Design review of the part built by this model. Coordinates are the model's own, in mm. Face numbers are marked on the shaded views. Coordinates: 2 decimals unless noted, no trailing zeros. Order: outer loops, then holes, each group sorted by start corner. A loop starts at its lowest first (then second) coordinate and runs counter-clockwise, first axis right, second up. Notation, with made-up numbers: (-32, 41) - (15, 41) arc R32 cw to (15, 77) - close; hole circle Ø1 at (52.25, 33). An arc over 180 degrees is marked (long way). Write each question's results on one line, items separated by ' | '. Start each with the question number.
```python
from build123d import *

# Parameters (mm, degrees)
SKETCH_1_R         = 30
SKETCH_1_R_2       = 23.5
EXTRUDE_1_DEPTH    = 10
SKETCH_2_R         = 31.5
SKETCH_2_R_2       = 30
EXTRUDE_2_DEPTH    = 2
HOLE_WIZARD_M4_1_D = 3.3


with BuildPart() as part:
    # 草图1 → 凸台-拉伸1 (new body)
    with BuildSketch(Plane(origin=(0, 0, 0), x_dir=(1, 0, 0), z_dir=(0, 1, 0))):
        Circle(SKETCH_1_R)
        Circle(SKETCH_1_R_2, mode=Mode.SUBTRACT)
    extrude(amount=EXTRUDE_1_DEPTH)

    # 草图2 → 凸台-拉伸2 (add)
    with BuildSketch(Plane(origin=(0, 10, 0), x_dir=(1, 0, 0), z_dir=(0, 1, 0))):
        Circle(SKETCH_2_R)
        Circle(SKETCH_2_R_2, mode=Mode.SUBTRACT)
    extrude(amount=-EXTRUDE_2_DEPTH)

    # M4 螺纹孔1 (through all)
    with Locations(Plane(origin=(-18.561553006, 0, 18.561553006), x_dir=(0, 0, -1), z_dir=(0, -1, 0))):
        with Locations((0, 0), (-7.688446994, 18.561553006), (18.561553006, -7.688446994), (37.123106012, 0), (44.811553006, 18.561553006), (37.123106012, 37.123106012), (18.561553006, 44.811553006), (0, 37.123106012)):
            Hole(HOLE_WIZARD_M4_1_D / 2)


solid = part.part
```
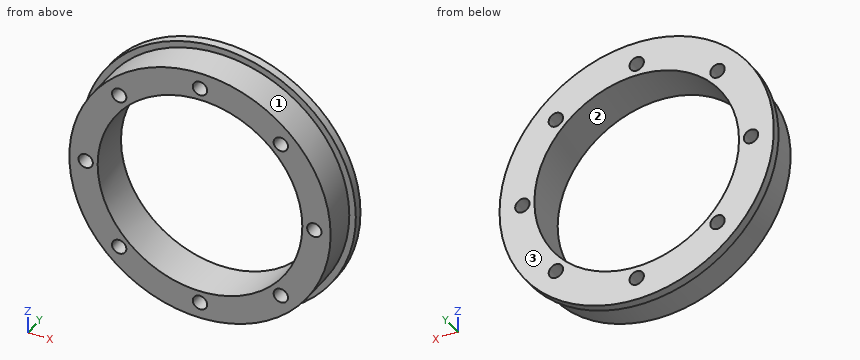
(1) Take a section at B-B (x = 0). State the section outline as (y, z) points.
(2) Mouldability with a two-part tool opening along Z and no side actions: class the marked faces 1, 2 and 3 as +Z half, -Z half, draft (parallel to the pull), parting line (faces both ways), or undercut.
(3) Clearance check with flat-ended pins moving along their axes: pin 1 (12 mm diameter, centred on x = 8.5, z = -16, fed in from +Y); pin 2 (6 mm diameter, centred on y = 2.5, z = -16.5, fed in from +X); pin 3 (6 mm diameter, centred on x = 10, y = 1, fed in from +Z); pin 4 (1 mm diameter, centred on x = 0.5, y = 5, fed in from -Z). State where each tip first meets the part, or that it passes through.
(4) Take a section at A-A (z = 0). State the section outline as (x, y) points.
(5) To check wall thickness, follow line 1 along X through (y, z) = (4.25, 0); line 2 along X through (y, z) = (2, -1); line 3 along X through (y, z) = (3.25, -21). State the ranges of each line that lie inside material, in increasing order. Write a range as [from, to].
(6) Take a section at D-D (z = -26.25). State the section outline as (x, y) points, plus the area to 3 significant figures.
(7) Take a section at C-C (x = -16). State the section outline as (y, z) points, plus the area to 3 significant figures.
Worked out:
1) outline: (0, -30) - (8, -30) - (8, -31.5) - (10, -31.5) - (10, -27.9) - (0, -27.9) - close; (0, -24.6) - (10, -24.6) - (10, -23.5) - (0, -23.5) - close; (0, 23.5) - (10, 23.5) - (10, 24.6) - (0, 24.6) - close; (0, 27.9) - (10, 27.9) - (10, 31.5) - (8, 31.5) - (8, 30) - (0, 30) - close
2) face 1: parting line | face 2: undercut | face 3: draft
3) pin 1: y = 10 | pin 2: x = 26.79 | pin 3: z = 29.17 | pin 4: z = -30
4) outline: (-31.5, 8) - (-30, 8) - (-30, 0) - (-27.9, 0) - (-27.9, 10) - (-31.5, 10) - close; (-24.6, 0) - (-23.5, 0) - (-23.5, 10) - (-24.6, 10) - close; (23.5, 0) - (24.6, 0) - (24.6, 10) - (23.5, 10) - close; (27.9, 0) - (30, 0) - (30, 8) - (31.5, 8) - (31.5, 10) - (27.9, 10) - close
5) line 1: [-30, -27.9], [-24.6, -23.5], [23.5, 24.6], [27.9, 30] | line 2: [-29.98, -27.56], [-24.94, -23.48], [23.48, 24.94], [27.56, 29.98] | line 3: [-21.42, -10.55], [10.55, 21.42]
6) outline: (-17.41, 8) - (-14.52, 8) - (-14.52, 0) - (-1.65, 0) - (-1.65, 10) - (-17.41, 10) - close; (1.65, 0) - (14.52, 0) - (14.52, 8) - (17.41, 8) - (17.41, 10) - (1.65, 10) - close | area: 269 mm^2
7) outline: (0, -25.38) - (8, -25.38) - (8, -27.13) - (10, -27.13) - (10, -17.21) - (0, -17.21) - close; (0, 17.21) - (10, 17.21) - (10, 27.13) - (8, 27.13) - (8, 25.38) - (0, 25.38) - close | area: 170 mm^2
